Design review of the part built by this model. Coordinates are the model's own, in mm. Face numbers are marked on the shaded views. Give positions to 0.01 mm unless a question says otherwise; leave off trailing zeros. Order: outer loops, then holes, each group sorted by start corner. A loop starts at its lowest first (then second) coordinate and runs counter-clockwise, first axis right, second up.
Autodesk Inventor part; units mm, degrees
ref_plane "YZ Plane" through (0, 0, 0) normal (1, 0, 0) x (0, 1, 0)
ref_plane "XZ Plane" through (0, 0, 0) normal (0, 1, 0) x (-1, 0, 0)
ref_plane "XY Plane" through (0, 0, 0) normal (0, 0, 1) x (1, 0, 0)
sketch "Sketch1" plane through (0, 0, 0) normal (0, 1, 0) x (-1, 0, 0)
  arc A0 (-7.9569, -0.8296) -> (7.9569, -0.8296) centre (0, 0) ccw
  line L0 (0, 0) -> (0, 67.5) construction
  arc A1 (14.9191, 65.9444) -> (-14.9191, 65.9444) centre (0, 67.5) ccw
  line L1 (14.9191, 65.9444) -> (7.9569, -0.8296)
  line L2 (-14.9191, 65.9444) -> (-7.9569, -0.8296)
  line L3 (8.9515, -0.9333) -> (15.9137, 65.8407)
  arc A2 (15.9137, 65.8407) -> (-15.9137, 65.8407) centre (0, 67.5) ccw
  line L4 (-15.9137, 65.8407) -> (-8.9515, -0.9333)
  arc A3 (-8.9515, -0.9333) -> (8.9515, -0.9333) centre (0, 0) ccw
  dimension "d0" = 16
  dimension "d1" = 67.5
  dimension "d2" = 30
  dimension "d3" = 1
extrude "Extrusion1" add sketch "Sketch1" along normal blind 8
properties part number "Belt"
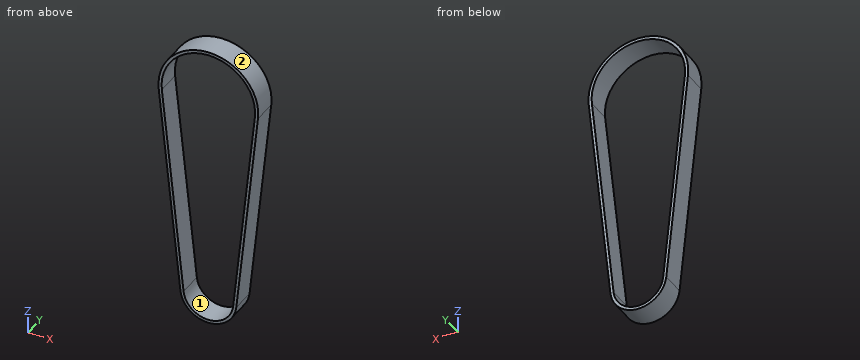
1. Draft analysis for pull direction X (two halves, no side actions). For the marked faces 1 and 2, state which applies: pulls with the +X half, pulls with the -X half, needs draft (parallel to the pull), parting line crosses it, or undercut.
Recorded:
face 1: undercut
face 2: parting line crosses it
2. Take a section at A-A (x = 0). State the section outline as (y, z) points, then the cut area to 3 significant figures.
Recorded:
outline: (0, -9) - (8, -9) - (8, -8) - (0, -8) - close; (0, 82.5) - (8, 82.5) - (8, 83.5) - (0, 83.5) - close
area: 16.0 mm2
3. Take a section at B-B (z = 67.5). State the section outline as (x, y) points.
Recorded:
outline: (-16, 0) - (-15, 0) - (-15, 8) - (-16, 8) - close; (15, 0) - (16, 0) - (16, 8) - (15, 8) - close
4. Take a section at C-C (y = 3.75). State the section outline as (x, z) points.
Recorded:
outline: (-15.91, 65.84) - (-8.95, -0.93) arc R9 ccw to (8.95, -0.93) - (15.91, 65.84) arc R16 ccw (long way) to start; hole (-14.92, 65.94) - (-7.96, -0.83) arc R8 ccw to (7.96, -0.83) - (14.92, 65.94) arc R15 ccw (long way) to start
5. For pin 1 (3 mm diameter, centred on y = 2.5, z = 15.5, fed in from +X); pin 2 (1.5 mm diameter, centred on y = 5.5, z = 74, fed in from +X); pin 3 (1.5 mm diameter, centred on y = 3, z = 51.5, fed in from +X), all flat-tipped, find the tip position at first contact; note any pin that passes through.
Recorded:
pin 1: stops at x = 10.82
pin 2: stops at x = 14.93
pin 3: stops at x = 14.5
6. For line 1 along X through (y, z) = (5, 67.5); line 2 along X through (y, z) = (4.25, 8); line 3 along Z through (x, y) = (3, 6), list the stretches that pass through material, from the lowest coordinate up.
Recorded:
line 1: x = -16 to -15, 15 to 16
line 2: x = -9.88 to -8.88, 8.88 to 9.88
line 3: z = -8.49 to -7.42, 82.2 to 83.22
